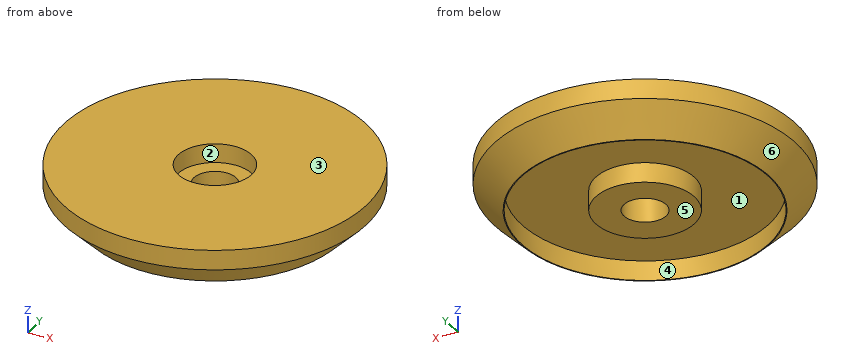
```python
from build123d import *

# Parameters (mm, degrees)
SKETCH2_R                = 17.181172962
BOSS_EXTRUDE1_DEPTH      = 1.25
BOSS_EXTRUDE1_DEPTH_BACK = 4
SKETCH3_R                = 14.079134115
SKETCH3_R_2              = 5.629774077
CUT_EXTRUDE1_DEPTH       = 2.25
SKETCH4_R                = 2.4
CUT_EXTRUDE2_DEPTH       = 12.25
SKETCH5_R                = 4.178678746
CUT_EXTRUDE3_DEPTH       = 2.15
CHAMFER1_SIZE            = 3
SCALE2_SCALE             = 0.75


with BuildPart() as part:
    # Sketch2 → Boss-Extrude1 (new body, two sides)
    with BuildSketch(Plane.XY.offset(-466.775167308)) as boss_extrude1_sk:
        Circle(SKETCH2_R)
    extrude(amount=BOSS_EXTRUDE1_DEPTH)
    extrude(boss_extrude1_sk.sketch, amount=-BOSS_EXTRUDE1_DEPTH_BACK)

    # Sketch3 → Cut-Extrude1 (cut)
    with BuildSketch(Plane(origin=(0, 0, -470.775167308), x_dir=(-1, 0, 0), z_dir=(0, 0, -1))):
        Circle(SKETCH3_R)
        Circle(SKETCH3_R_2, mode=Mode.SUBTRACT)
    extrude(amount=-CUT_EXTRUDE1_DEPTH, mode=Mode.SUBTRACT)

    # Sketch4 → Cut-Extrude2 (cut)
    with BuildSketch(Plane(origin=(0, 0, -470.775167308), x_dir=(-1, 0, 0), z_dir=(0, 0, -1))):
        Circle(SKETCH4_R)
    extrude(amount=-CUT_EXTRUDE2_DEPTH, mode=Mode.SUBTRACT)

    # Sketch5 → Cut-Extrude3 (cut)
    with BuildSketch(Plane.XY.offset(-465.525167308)):
        Circle(SKETCH5_R)
    extrude(amount=-CUT_EXTRUDE3_DEPTH, mode=Mode.SUBTRACT)

    # Chamfer1
    chamfer1_edges = [part.edges().sort_by_distance(p)[0] for p in [
        (-17.181172962, 0, -470.775167308),
    ]]
    chamfer(chamfer1_edges, length=CHAMFER1_SIZE)


with BuildPart() as part_1:
    # Scale2: scaled about (0, 0, -467.372549258)
    add(part.part.scale(SCALE2_SCALE).moved(Location((0, 0, -116.843137314))))


solid = part_1.part
```
The model under review builds one solid part; all positions refer to its coordinate system, in mm. Face numbers are marked on the shaded views. A direction names the side the tool comes from. Round coordinates to 2 decimals unless told otherwise and drop trailing zeros. Loops run counter-clockwise (first coordinate to the right, second up) from the corner with the lowest first, then second, coordinate; pieces in that order, holes last. Notation, with made-up numbers: (-11.5, 45.25) -> (43.5, 45.25) arc R25 cw to (43.5, 72.25) -> close; hole circle Ø3 at (46.5, 88). An arc over 180 degrees is marked (long way). Answer in a Markdown table with one row per item.
1) Consider section A-A, the plane y = 0. Write out the cut boundary in (x, z), plus the area to 3 significant figures.
Taken from the geometry:
| item | result |
|---|---|
| outline | (-12.89, -467.67) -> (-10.64, -469.92) -> (-10.56, -469.92) -> (-10.56, -468.24) -> (-4.22, -468.24) -> (-4.22, -469.92) -> (-1.8, -469.92) -> (-1.8, -467.6) -> (-3.13, -467.6) -> (-3.13, -465.99) -> (-12.89, -465.99) -> close; (1.8, -469.92) -> (4.22, -469.92) -> (4.22, -468.24) -> (10.56, -468.24) -> (10.56, -469.92) -> (10.64, -469.92) -> (12.89, -467.67) -> (12.89, -465.99) -> (3.13, -465.99) -> (3.13, -467.6) -> (1.8, -467.6) -> close |
| area | 56.5 mm² |
2) Draft analysis for pull direction Y (two halves, no side actions). For the marked faces 4, 5 and 6, state which applies: pulls with the +Y half, pulls with the -Y half, needs draft (parallel to the pull), parting line crosses it, or undercut.
Taken from the geometry:
| item | result |
|---|---|
| face 4 | undercut |
| face 5 | needs draft |
| face 6 | parting line crosses it |
3) Tool access review of the marked faces 1, 2 and 3: name each direction out of +Z, -Z, +X, -X, +Y, -Y from which nothing blocks a thin tool from reaching the whole face with its end or side.
Taken from the geometry:
| item | result |
|---|---|
| face 1 | -Z |
| face 2 | +Z |
| face 3 | +Z, +X, -X, +Y, -Y |
4) Consider section D-D, the plane z = -466.3. Write out the cut boundary in (x, y).
Taken from the geometry:
| item | result |
|---|---|
| outline | circle Ø25.77 at (0, 0); hole circle Ø6.27 at (0, 0) |
5) Consider section C-C, the plane z = -469.4. Write out the cut boundary in (x, y), plus the area to 3 significant figures.
Taken from the geometry:
| item | result |
|---|---|
| outline | circle Ø22.32 at (0, 0); circle Ø8.44 at (0, 0); hole circle Ø21.12 at (0, 0); hole circle Ø3.6 at (0, 0) |
| area | 86.8 mm² |
6) For pin 1 Ø3 at (x, y) = (0, 0) entering from -Z; pin 2 Ø2 at (x, z) = (6, -467.5) entering from -Y; pin 3 Ø1.9 at (x, y) = (-1.5, -1.5) entering from +Z, all flat-tipped, find the tip position at first contact; note any pin that passes through.
Taken from the geometry:
| item | result |
|---|---|
| pin 1 | passes through |
| pin 2 | stops at y = -11.88 |
| pin 3 | stops at z = -467.6 |
7) Wall thickness on line 1 along Y through (x, z) = (-0.75, -469.3); line 2 along Z through (x, y) = (-8.5, -5.5); line 3 along Y through (x, z) = (0, -469.4): over which ranges is each line inside the solid? List them lowest first.
Taken from the geometry:
| item | result |
|---|---|
| line 1 | y = -11.24 to -10.53, -4.16 to -1.64, 1.64 to 4.16, 10.53 to 11.24 |
| line 2 | z = -468.24 to -465.99 |
| line 3 | y = -11.16 to -10.56, -4.22 to -1.8, 1.8 to 4.22, 10.56 to 11.16 |
